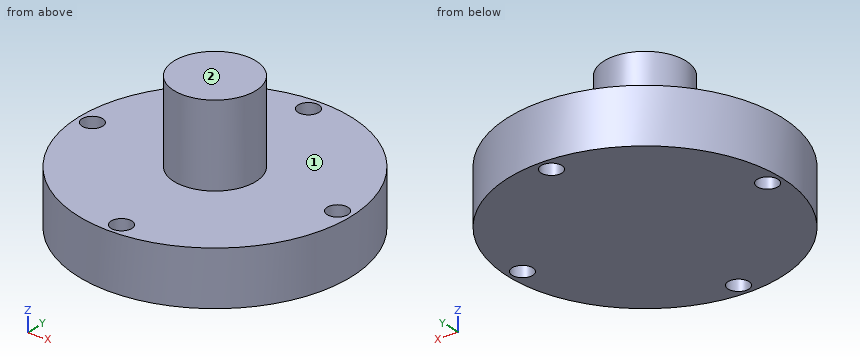
```python
from build123d import *

# Parameters (mm, degrees)
F3_D            = 4.826
F3_COPIES_COUNT = 4


# Not quite as in the source:
# - a pattern or mirror of a feature is missing from the dataset's text; its kind, count and spacing are read off the source's solid


with BuildPart() as f1:
    # F0 (on Front) → F1 (revolve)
    with BuildSketch(Plane.XZ):
        Polygon((-31.75, 0), (0, 0), (0, 31.75), (-9.525, 31.75), (-9.525, 12.7), (-31.75, 12.7), align=None)
    revolve(axis=Axis((0, 0, 15.875), (0, 0, -1)))

    # F3 (through all)
    with Locations(Plane.XY.offset(12.7)):
        with Locations((0, 28.448)):
            f3 = Hole(F3_D / 2)

    # F3_copies: F3 ×4 about axis
    f3_copies_axis = Axis((0, 0, 0), (0, 0, 1))
    for i in range(1, F3_COPIES_COUNT):
        add(f3.rotate(f3_copies_axis, i * 360 / F3_COPIES_COUNT), mode=Mode.SUBTRACT)


solid = f1.part
```
The model under review builds one solid part; all positions refer to its coordinate system, in mm. Face numbers are marked on the shaded views. A direction names the side the tool comes from. Round coordinates to 2 decimals unless told otherwise and drop trailing zeros. Loops run counter-clockwise (first coordinate to the right, second up) from the corner with the lowest first, then second, coordinate; pieces in that order, holes last. Notation, with made-up numbers: (-29, 14.5) -> (12, 14.5) arc R4 cw to (12, 19.5) -> close; hole circle Ø8 at (17, 89). An arc over 180 degrees is marked (long way). Answer in a Markdown table with one row per item.
1) Tool access review of the marked faces 1 and 2: name each direction out of +Z, -Z, +X, -X, +Y, -Y from which nothing blocks a thin tool from reaching the whole face with its end or side.
Taken from the geometry:
| item | result |
|---|---|
| face 1 | +Z |
| face 2 | +Z, +X, -X, +Y, -Y |
2) Wall thickness on line 1 along Y through (x, z) = (0, 4.5) (3 decimals); line 2 along Z through (x, y) = (28, -9); line 3 along Y through (x, z) = (-7.5, 9.5): over which ranges is each line inside the solid? List them lowest first.
Taken from the geometry:
| item | result |
|---|---|
| line 1 | y = -31.75 to -30.861, -26.035 to 26.035, 30.861 to 31.75 |
| line 2 | z = 0 to 12.7 |
| line 3 | y = -30.85 to 30.85 |
3) Consider section D-D, the plane y = -6.5. Write out the cut boundary in (x, z), plus the area to 3 significant figures.
Taken from the geometry:
| item | result |
|---|---|
| outline | (-31.08, 0) -> (31.08, 0) -> (31.08, 12.7) -> (6.96, 12.7) -> (6.96, 31.75) -> (-6.96, 31.75) -> (-6.96, 12.7) -> (-31.08, 12.7) -> close |
| area | 1,050 mm² |
4) Consider section C-C, the plane z = 11. Write out the cut boundary in (x, y), plus the area to 3 significant figures.
Taken from the geometry:
| item | result |
|---|---|
| outline | circle Ø63.5 at (0, 0); hole circle Ø4.83 at (-28.45, 0); hole circle Ø4.83 at (0, -28.45); hole circle Ø4.83 at (0, 28.45); hole circle Ø4.83 at (28.45, 0) |
| area | 3,090 mm² |
5) Consider section A-A, the plane x = 0. Write out the cut boundary in (y, z) (3 decimals), plus the area to 3 significant figures.
Taken from the geometry:
| item | result |
|---|---|
| outline | (-31.75, 0) -> (-30.861, 0) -> (-30.861, 12.7) -> (-31.75, 12.7) -> close; (-26.035, 0) -> (26.035, 0) -> (26.035, 12.7) -> (9.525, 12.7) -> (9.525, 31.75) -> (-9.525, 31.75) -> (-9.525, 12.7) -> (-26.035, 12.7) -> close; (30.861, 0) -> (31.75, 0) -> (31.75, 12.7) -> (30.861, 12.7) -> close |
| area | 1,050 mm² |
6) For pin 1 Ø7.5 at (x, y) = (0, -28.448) entering from +Z; pin 2 Ø12 at (y, z) = (17.5, 13) entering from -X; pin 3 Ø2 at (x, z) = (-6.5, 20) entering from -Y; pin 4 Ø10 at (x, y) = (-24.5, -0.5) entering from -Z, all flat-tipped, find the tip position at first contact; note any pin that passes through.
Taken from the geometry:
| item | result |
|---|---|
| pin 1 | stops at z = 12.7 |
| pin 2 | stops at x = -29.59 |
| pin 3 | stops at y = -7.78 |
| pin 4 | stops at z = 0 |
